Can you work these out from the model? Positions are in its coordinate system, mm. A direction names the side the tool comes from. Give positions to 0.01 mm unless a question says otherwise; leave off trailing zeros. Loops run counter-clockwise (first coordinate to the right, second up) from the corner with the lowest first, then second, coordinate; pieces in that order, holes last. Notation, with made-up numbers: M 51.5,69.5 L 88.5,69.5 A31 ccw 88.5,97.5 Z; hole C 31,-37 d7. An arc over 180 degrees is marked long. Use CSV: the item, a comma, the result in double quotes.
from build123d import *

# Parameters (mm, degrees)
F1_DEPTH = 260
F2_DEPTH = 260
F0_W     = 1050
F0_H     = 180
F3_DEPTH = 260
F4_DEPTH = 1490
F5_DEPTH = 460


with BuildPart() as f1:
    # F0 (on Front) → F1 (new body)
    with BuildSketch(Plane.XZ):
        with BuildLine():
            Line((-519.379077, -442.715838), (5.620923, -442.715838))
            Line((5.620923, -442.715838), (530.620923, -442.715838))
            add(Edge.make_bspline(
                [(530.620923, -442.715838), (552.28759, -286.049171), (547.647588, 27.284162), (595.620923, 27.284162)],
                knots=[0, 0, 0, 0, 474.473392, 474.473392, 474.473392, 474.473392], degree=3))
            add(Edge.make_bspline(
                [(595.620923, 27.284162), (584.550135, 154.130891), (591.930621, 434.590191), (530.620923, 437.284162)],
                knots=[0, 0, 0, 0, 415.120464, 415.120464, 415.120464, 415.120464], degree=3))
            add(Edge.make_bspline(
                [(530.620923, 437.284162), (484.913282, 456.731707), (173.086815, 456.731707), (5.620923, 457.284162)],
                knots=[0, 0, 0, 0, 525.380814, 525.380814, 525.380814, 525.380814], degree=3))
            add(Edge.make_bspline(
                [(-519.379077, 437.284162), (-473.671436, 456.731707), (-161.844969, 456.731707), (5.620923, 457.284162)],
                knots=[0, 0, 0, 0, 525.380814, 525.380814, 525.380814, 525.380814], degree=3))
            add(Edge.make_bspline(
                [(-584.379077, 27.284162), (-573.308289, 154.130891), (-580.688775, 434.590191), (-519.379077, 437.284162)],
                knots=[0, 0, 0, 0, 415.120464, 415.120464, 415.120464, 415.120464], degree=3))
            add(Edge.make_bspline(
                [(-519.379077, -442.715838), (-541.045744, -286.049171), (-536.405742, 27.284162), (-584.379077, 27.284162)],
                knots=[0, 0, 0, 0, 474.473392, 474.473392, 474.473392, 474.473392], degree=3))
        make_face()
    extrude(amount=-F1_DEPTH)

    # F0 (on Front) → F2 (join)
    with BuildSketch(Plane.XZ):
        Polygon((530.620923, -442.715838), (5.620923, -442.715838), (-519.379077, -442.715838), (-519.379077, -552.715838), (530.620923, -552.715838), align=None)
    extrude(amount=-F2_DEPTH)

    # F0 (on Front) → F3 (join)
    with BuildSketch(Plane.XZ):
        with Locations((5.620923, -642.715838)):
            Rectangle(F0_W, F0_H)
    extrude(amount=-F3_DEPTH)

    # F0 (on Front) → F4 (join)
    with BuildSketch(Plane.XZ):
        with BuildLine():
            Line((-519.379077, -442.715838), (5.620923, -442.715838))
            Line((5.620923, -442.715838), (530.620923, -442.715838))
            add(Edge.make_bspline(
                [(530.620923, -442.715838), (552.28759, -286.049171), (547.647588, 27.284162), (595.620923, 27.284162)],
                knots=[0, 0, 0, 0, 474.473392, 474.473392, 474.473392, 474.473392], degree=3))
            add(Edge.make_bspline(
                [(595.620923, 27.284162), (584.550135, 154.130891), (591.930621, 434.590191), (530.620923, 437.284162)],
                knots=[0, 0, 0, 0, 415.120464, 415.120464, 415.120464, 415.120464], degree=3))
            add(Edge.make_bspline(
                [(530.620923, 437.284162), (484.913282, 456.731707), (173.086815, 456.731707), (5.620923, 457.284162)],
                knots=[0, 0, 0, 0, 525.380814, 525.380814, 525.380814, 525.380814], degree=3))
            add(Edge.make_bspline(
                [(-519.379077, 437.284162), (-473.671436, 456.731707), (-161.844969, 456.731707), (5.620923, 457.284162)],
                knots=[0, 0, 0, 0, 525.380814, 525.380814, 525.380814, 525.380814], degree=3))
            add(Edge.make_bspline(
                [(-584.379077, 27.284162), (-573.308289, 154.130891), (-580.688775, 434.590191), (-519.379077, 437.284162)],
                knots=[0, 0, 0, 0, 415.120464, 415.120464, 415.120464, 415.120464], degree=3))
            add(Edge.make_bspline(
                [(-519.379077, -442.715838), (-541.045744, -286.049171), (-536.405742, 27.284162), (-584.379077, 27.284162)],
                knots=[0, 0, 0, 0, 474.473392, 474.473392, 474.473392, 474.473392], degree=3))
        make_face()
    extrude(amount=F4_DEPTH)

    # F0 (on Front) → F5 (join)
    with BuildSketch(Plane.XZ):
        Polygon((530.620923, -442.715838), (5.620923, -442.715838), (-519.379077, -442.715838), (-519.379077, -552.715838), (530.620923, -552.715838), align=None)
    extrude(amount=F5_DEPTH)


solid = f1.part
Q1. I want a section at B-B, the plane z = -477.5. Please give me the cut outline in (x, y).
Model answer:
outline,"M -519.38,-460 L 530.62,-460 L 530.62,260 L -519.38,260 Z"
Q2. For faces 1 (the flat face through (530.621, -15, -525)), 2 (the flat face through (-519.379, -15, -521)), 3 (the flat face through (-2, -460, -497)), which set-ups out of +Z, -Z, +X, -X, +Y, -Y let a thin tool reach every point of the face, with its end or its side?
Model answer:
face 1,"-Z, +X, +Y, -Y"
face 2,"-Z, -X, +Y, -Y"
face 3,"-Z, +X, -X, -Y"
Q3. Please list where these lines run through material, in increasing order: L1, parallel to Z at x = -57, y = -551; L2, parallel to Z at x = 120.5, y = -734; L3, parallel to Y at x = -50.5, z = -557. Write a range as from..to.
Model answer:
L1,"-442.72..457.09"
L2,"-442.72..456.86"
L3,"0..260"
Q4. I'm going to push flat-ended pins straight in: P1, Ø2, axis at x = -444, y = -381.5, coming from the -Z side; P2, Ø2, axis at y = -127.5, z = -33, coming from the +X side; P3, Ø1, axis at x = -95, y = -492, coming from the -Z side. Where does each tip first touch, or does it pass through?
Model answer:
P1,"z = -552.72"
P2,"x = 566.71"
P3,"z = -442.72"
Q5. I want a section at A-A, the plane z = -655.5. Please give me the cut outline in (x, y).
Model answer:
outline,"M -519.38,0 L 530.62,0 L 530.62,260 L -519.38,260 Z"
